Input: part model. Units: mm. Frame: model coordinates. A direction names the side the tool comes from. Round coordinates to 2 decimals unless told otherwise and drop trailing zeros. Loops run counter-clockwise (first coordinate to the right, second up) from the corner with the lowest first, then second, coordinate; pieces in that order, holes last. Notation, with made-up numbers: M 20.5,34 L 40.5,34 A19 ccw 40.5,57 Z; hole C 42,83 d11. An arc over 180 degrees is marked long. Put each result on its own line as item: value. Start each with the question number.
1) Section A-A on y = 0. Output: boundary loops of the cut face in (x, z), plus the area to 3 significant figures.
2) Reachability of faces 4 (the face through (58.3, 147.093, 11.339)), 5 (the face through (-75.815, -96.921, 18.437)) from +Z, -Z, +X, -X, +Y, -Y: full face, straight path, thin tool, end or side. Return the list, or none.
3) Section B-B on x = -51.5. Output: boundary loops of the cut face in (y, z).
4) Line query: probe 1 along X at (y, z) = (-112.5, 5.5); probe 2 along Y at (x, z) = (23, 3.5); probe 3 along X at (y, z) = (-22, 10). Output: solid intervals per line, ascending.
5) Section C-C on y = 67. Output: boundary loops of the cut face in (x, z).
6) Pin query (flat end, axial travel): pin 1 (1 mm diameter, centred on x = -83, z = 17, fed in from +Y); pin 2 (11 mm diameter, centred on x = -116.54, y = -104.96, fed in from +Z); pin 3 (4 mm diameter, centred on x = -41, z = 4.5, fed in from -Y). Return the tip coordinate at first contact, or that it passes through.
7) Draft query along Y for faces 1 (the face through (86.349, 106.868, 11.339)), 2 (the face through (126.715, -42.843, 5.423)), 3 (the face through (105.38, -126.29, 11.34)). Return one class per face: +Y half, -Y half, draft (parallel to the pull), parting line (faces both ways), or undercut.
from build123d import *

# Parameters (mm, degrees)
BOSS_EXTRUDE1_DEPTH             = 23
FILLET2_R                       = 50.8
SKETCH2_R                       = 40.05
CUT_EXTRUDE1_DEPTH              = 16
SKETCH5_R                       = 36.83
CUT_EXTRUDE2_DEPTH              = 25.4
FILLET5_R                       = 1
FILLET6_R                       = 1
CBORE_FOR_M10_SHCS7_D           = 10.5
CBORE_FOR_M10_SHCS7_CBORE_D     = 18
CBORE_FOR_M10_SHCS7_CBORE_DEPTH = 12
TAP_DRILL_FOR_M8X1_25_TAP2_D    = 6.8
F_8_0MM_DOWEL_HOLE1_D           = 8
F_8_0MM_DOWEL_HOLE1_DEPTH       = 9
F_8_0MM_DOWEL_HOLE1_TIP         = 2.403442476
F_10_0MM_DOWEL_HOLE3_D          = 10
F_10_0MM_DOWEL_HOLE3_DEPTH      = 10
F_10_0MM_DOWEL_HOLE3_TIP        = 3.004303095
CBORE_FOR_M10_SHCS9_D           = 10.5
CBORE_FOR_M10_SHCS9_CBORE_D     = 18
CBORE_FOR_M10_SHCS9_CBORE_DEPTH = 10


with BuildPart() as part:
    # Sketch1 → Boss-Extrude1 (new body)
    with BuildSketch(Plane.XY):
        with BuildLine():
            Line((84.221105008, -163.490124242), (2.699306526, -136.831626991))
            Line((2.699306526, -136.831626991), (-67.458438584, -162.730244564))
            ThreePointArc((-67.458438584, -162.730244564), (-75.680634631, -163.297391653), (-82.910842941, -159.341351783))
            Line((-82.910842941, -159.341351783), (-126.914053579, -115.336397895))
            ThreePointArc((-126.914053579, -115.336397895), (-130.093640928, -110.577690662), (-131.210211433, -104.964461595))
            Line((-131.210211433, -104.964461595), (-131.213297338, 125.035476514))
            ThreePointArc((-131.213297338, 125.035476514), (-126.350161673, 135.869915187), (-115.02264263, 139.436771249))
            Line((-115.02264263, 139.436771249), (-20.796830867, 128.37488637))
            Line((-20.796830867, 128.37488637), (49.24312976, 147.55277548))
            ThreePointArc((49.24312976, 147.55277548), (58.421803723, 147.044752766), (65.450410839, 141.119820294))
            Line((65.450410839, 141.119820294), (107.841002341, 71.642808501))
            ThreePointArc((107.841002341, 71.642808501), (117.701476238, 53.952608996), (124.683759391, 34.941564155))
            Line((124.683759391, 34.941564155), (145.845410308, -40.455794779))
            ThreePointArc((145.845410308, -40.455794779), (145.61886709, -49.11646402), (140.544799405, -56.138739339))
            Line((140.544799405, -56.138739339), (109.149264581, -79.773969292))
            Line((109.149264581, -79.773969292), (103.401152517, -150.732337669))
            ThreePointArc((103.401152517, -150.732337669), (96.90432541, -161.761540655), (84.221105008, -163.490124242))
        make_face()
    extrude(amount=BOSS_EXTRUDE1_DEPTH)

    # Fillet2
    fillet2_edges = [part.edges().sort_by_distance(p)[0] for p in [
        (109.149264581, -79.773969292, 11.5),
        (2.699306526, -136.831626991, 11.5),
        (-20.796830867, 128.37488637, 11.5),
    ]]
    fillet(fillet2_edges, radius=FILLET2_R)

    # Sketch2 → Cut-Extrude1 (cut)
    with BuildSketch(Plane(origin=(0, 0, 23), x_dir=(-1, 0, 0), z_dir=(0, 0, -1))):
        Circle(SKETCH2_R)
    extrude(amount=CUT_EXTRUDE1_DEPTH, mode=Mode.SUBTRACT)

    # Sketch5 → Cut-Extrude2 (cut)
    with BuildSketch(Plane(origin=(0, 0, 23), x_dir=(-1, 0, 0), z_dir=(0, 0, -1))):
        Circle(SKETCH5_R)
    extrude(amount=CUT_EXTRUDE2_DEPTH, mode=Mode.SUBTRACT)

    # Fillet5
    fillet5_edges = [part.edges().sort_by_distance(p)[0] for p in [
        (40.05, 0, 23),
    ]]
    fillet(fillet5_edges, radius=FILLET5_R)

    # Fillet6
    fillet6_edges = [part.edges().sort_by_distance(p)[0] for p in [
        (40.05, 0, 7),
    ]]
    fillet(fillet6_edges, radius=FILLET6_R)

    # CBORE for M10 SHCS7 (through all)
    with Locations(Plane.XY.offset(23)):
        with Locations((-116.713297339, 125.03567106), (-116.541509562, -104.964264785), (-72.538298924, -148.969218673), (53.072470058, 133.567563544), (131.722431635, -44.419667636), (88.780343848, -149.547952394)):
            CounterBoreHole(CBORE_FOR_M10_SHCS7_D / 2, CBORE_FOR_M10_SHCS7_CBORE_D / 2, CBORE_FOR_M10_SHCS7_CBORE_DEPTH)

    # Tap Drill for M8x1.25 Tap2 (through all)
    with Locations(Plane.XY.offset(23)):
        with Locations((46, 97.92), (-31, 98), (-105.616623552, 111.626092354), (-105.616623552, -112.292869781), (-31.12, -98.35), (45.85, -98.52), (78.925, -30.46), (77.9, 39.75)):
            Hole(TAP_DRILL_FOR_M8X1_25_TAP2_D / 2)

    # Ø8.0mm Dowel Hole1
    with Locations(Plane.XY.offset(23)):
        with Locations((-72, 97.977867106), (-72, -98.122132894)):
            Hole(F_8_0MM_DOWEL_HOLE1_D / 2, depth=F_8_0MM_DOWEL_HOLE1_DEPTH)
            with Locations((0, 0, -(F_8_0MM_DOWEL_HOLE1_DEPTH + F_8_0MM_DOWEL_HOLE1_TIP / 2))):  # 118° drill point
                Cone(0, F_8_0MM_DOWEL_HOLE1_D / 2, F_8_0MM_DOWEL_HOLE1_TIP, mode=Mode.SUBTRACT)

    # Ø10.0mm Dowel Hole3
    with Locations(Plane(origin=(0, 0, 0), x_dir=(-1, 0, 0), z_dir=(0, 0, -1))):
        with Locations((76.55340813, 103.753913834), (-59.102558089, -114.980445858)):
            Hole(F_10_0MM_DOWEL_HOLE3_D / 2, depth=F_10_0MM_DOWEL_HOLE3_DEPTH)
            with Locations((0, 0, -(F_10_0MM_DOWEL_HOLE3_DEPTH + F_10_0MM_DOWEL_HOLE3_TIP / 2))):  # 118° drill point
                Cone(0, F_10_0MM_DOWEL_HOLE3_D / 2, F_10_0MM_DOWEL_HOLE3_TIP, mode=Mode.SUBTRACT)

    # CBORE for M10 SHCS9 (through all)
    with Locations(Plane.XY.offset(23)):
        with Locations((53.072470058, 133.567563544), (131.722431635, -44.419667636), (88.780343848, -149.547952394), (-116.713297339, 125.03567106), (-116.541509562, -104.964264785), (-72.538298924, -148.969218673)):
            CounterBoreHole(CBORE_FOR_M10_SHCS9_D / 2, CBORE_FOR_M10_SHCS9_CBORE_D / 2, CBORE_FOR_M10_SHCS9_CBORE_DEPTH)


solid = part.part
Geometry results:
1. outline: M -131.21,0 L -36.83,0 L -36.83,7 L -39.05,7 A1 cw -40.05,8 L -40.05,22 A1 ccw -41.05,23 L -131.21,23 Z; M 36.83,0 L 134.49,0 L 134.49,23 L 41.05,23 A1 ccw 40.05,22 L 40.05,8 A1 cw 39.05,7 L 36.83,7 Z
1. area: 4,310 mm²
2. face 4: +Z, -Z, +Y
2. face 5: +Z
3. outline: M -156.84,0 L 131.98,0 L 131.98,23 L -156.84,23 Z
4. probe 1: x = -129.13 to -109.01, -102.22 to 54.76, 63.44 to 106.5
4. probe 2: y = -143.47 to -28.77, 28.77 to 140.37
4. probe 3: x = -131.21 to -33.47, 33.47 to 140.67
5. outline: M -131.21,0 L 110.79,0 L 110.79,23 L -131.21,23 Z
6. pin 1: stops at y = 135.74
6. pin 2: stops at z = 11
6. pin 3: stops at y = -153.7
7. face 1: +Y half
7. face 2: undercut
7. face 3: -Y half
